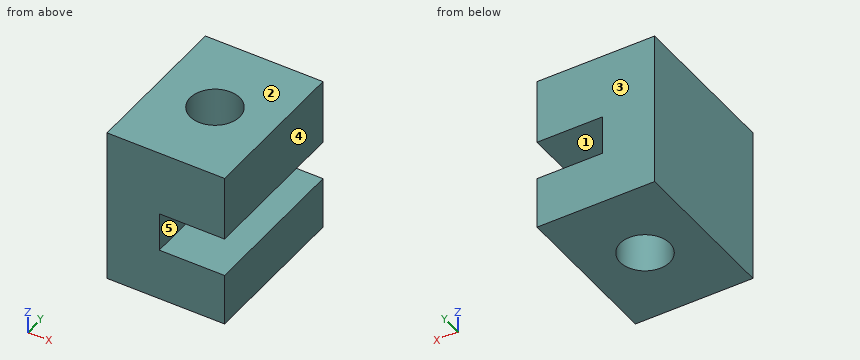
```python
from build123d import *

# Parameters (mm, degrees)
SKETCH1_W           = 5
SKETCH1_H           = 5
BOSS_EXTRUDE2_DEPTH = 6
SKETCH2_R           = 1.9
CUT_EXTRUDE1_DEPTH  = 13


with BuildPart() as part:
    # Sketch1 → Boss-Extrude2 (new body, symmetric)
    with BuildSketch(Plane(origin=(0, 0, 0), x_dir=(1, 0, 0), z_dir=(0, 1, 0))):
        Polygon((-4.5, 6), (-4.5, -6), (-0.5, -6), (-0.5, -1), (-0.5, 2), (4.5, 2), (4.5, 6), align=None)
        with Locations((2, -3.5)):
            Rectangle(SKETCH1_W, SKETCH1_H)
    extrude(amount=BOSS_EXTRUDE2_DEPTH, both=True)

    # Sketch2 → Cut-Extrude1 (cut, through all)
    with BuildSketch(Plane(origin=(0, 0, -6), x_dir=(-1, 0, 0), z_dir=(0, 0, -1))):
        Circle(SKETCH2_R)
    extrude(amount=-CUT_EXTRUDE1_DEPTH, mode=Mode.SUBTRACT)


solid = part.part
```
Geometry check sheet. Reference: the model listing, model coordinates, mm. Face numbers are marked on the shaded views. A direction names the side the tool comes from. Round coordinates to 2 decimals unless told otherwise and drop trailing zeros. Order: outer loops, then holes, each group sorted by start corner. A loop starts at its lowest first (then second) coordinate and runs counter-clockwise, first axis right, second up. Notation, with made-up numbers: (4.5, -16) - (60.5, -16) arc R15 cw to (60.5, 9) - close; hole circle Ø9 at (35.5, 88.25). An arc over 180 degrees is marked (long way). Use a Markdown table: item, result. Add a question column.
1) Section check C-C (y = -0.5). Record the cut outline in (x, z).
2) Mould release check, pull along Z, two halves, no side actions. Record for the marked faces 1, 2 and 3: released by +Z, released by -Z, zero draft, split by the parting line, or undercut.
3) Section check D-D (z = -2.25). Record the cut outline in (x, y), then the cut area to 3 significant figures.
4) Gauge pin test, flat ends, axial feed: P1, Ø2.5, axis at x = 0, y = 0, coming from the +Z side; P2, Ø0.9, axis at y = -4.5, z = -0.5, coming from the +X side. Record the tip position at first contact, or that the pin passes through.
5) Thickness scan on line 1 along Z through (x, y) = (3, -2); line 2 along X through (y, z) = (0, 2); line 3 along Y through (x, z) = (0, -2.75). Record the ranges inside material, lowest first.
6) Section check B-B (x = 3). Record the cut outline in (y, z).
7) Set-up check for the marked faces 4 and 5: record each of +Z, -Z, +X, -X, +Y, -Y from which the full face is reachable in a straight line by a thin tool's end or side.
8) Section check A-A (x = 0). Record the cut outline in (y, z).
Established:
| question | item | result |
|---|---|---|
| 1 | outline | (-4.5, -6) - (-1.83, -6) - (-1.83, 6) - (-4.5, 6) - close; (1.83, -6) - (4.5, -6) - (4.5, -2) - (1.83, -2) - close; (1.83, 1) - (4.5, 1) - (4.5, 6) - (1.83, 6) - close |
| 2 | face 1 | undercut |
| 2 | face 2 | released by +Z |
| 2 | face 3 | zero draft |
| 3 | outline | (-4.5, -6) - (4.5, -6) - (4.5, 6) - (-4.5, 6) - close; hole circle Ø3.8 at (0, 0) |
| 3 | area | 96.7 mm2 |
| 4 | P1 | through |
| 4 | P2 | x = -0.5 |
| 5 | line 1 | -6 to -2, 1 to 6 |
| 5 | line 2 | -4.5 to -1.9, 1.9 to 4.5 |
| 5 | line 3 | -6 to -1.9, 1.9 to 6 |
| 6 | outline | (-6, -6) - (6, -6) - (6, -2) - (-6, -2) - close; (-6, 1) - (6, 1) - (6, 6) - (-6, 6) - close |
| 7 | face 4 | +Z, -Z, +X, +Y, -Y |
| 7 | face 5 | +X, +Y, -Y |
| 8 | outline | (-6, -6) - (-1.9, -6) - (-1.9, -2) - (-6, -2) - close; (-6, 1) - (-1.9, 1) - (-1.9, 6) - (-6, 6) - close; (1.9, -6) - (6, -6) - (6, -2) - (1.9, -2) - close; (1.9, 1) - (6, 1) - (6, 6) - (1.9, 6) - close |
